Here's how the part is built. I have some questions about the finished solid (model axes, mm). A direction names the side the tool comes from. Give positions to 0.01 mm unless a question says otherwise; leave off trailing zeros. Loops run counter-clockwise (first coordinate to the right, second up) from the corner with the lowest first, then second, coordinate; pieces in that order, holes last. Notation, with made-up numbers: (19, 56.5) - (42, 56.5) arc R10 ccw to (42, 74.5) - close; hole circle Ø6 at (59, -12.5). An arc over 180 degrees is marked (long way). Use a Markdown table: item, result.
from build123d import *

# Parameters (mm, degrees)
SKETCH_1_W          = 42
SKETCH_1_H          = 42
EXTRUDE_1_DEPTH     = 5
SKETCH_2_R          = 17.5
CUT_EXTRUDE_1_DEPTH = 6
SKETCH_3_R          = 18.5
CUT_EXTRUDE_2_DEPTH = 4
SKETCH_4_R          = 19
CUT_EXTRUDE_3_DEPTH = 2
FILLET_1_R          = 4
SKETCH_5_R          = 1.6
CUT_EXTRUDE_4_DEPTH = 6
SKETCH_7_R          = 1.15
CUT_EXTRUDE_5_DEPTH = 6
SKETCH_8_R          = 2
CUT_EXTRUDE_6_DEPTH = 3


with BuildPart() as part:
    # 草图1 → 凸台-拉伸1 (new body)
    with BuildSketch(Plane.XY):
        Rectangle(SKETCH_1_W, SKETCH_1_H)
    extrude(amount=EXTRUDE_1_DEPTH)

    # 草图2 → 切除-拉伸1 (cut, through all)
    with BuildSketch(Plane.XY.offset(5)):
        Circle(SKETCH_2_R)
    extrude(amount=-CUT_EXTRUDE_1_DEPTH, mode=Mode.SUBTRACT)

    # 草图3 → 切除-拉伸2 (cut)
    with BuildSketch(Plane.XY.offset(5)):
        Circle(SKETCH_3_R)
    extrude(amount=-CUT_EXTRUDE_2_DEPTH, mode=Mode.SUBTRACT)

    # 草图4 → 切除-拉伸3 (cut)
    with BuildSketch(Plane.XY.offset(5)):
        Circle(SKETCH_4_R)
    extrude(amount=-CUT_EXTRUDE_3_DEPTH, mode=Mode.SUBTRACT)

    # 圆角1
    fillet_1_edges = [part.edges().sort_by_distance(p)[0] for p in [
        (21, -21, 2.5),
        (-21, -21, 2.5),
        (-21, 21, 2.5),
        (21, 21, 2.5),
    ]]
    fillet(fillet_1_edges, radius=FILLET_1_R)

    # 草图5 → 切除-拉伸4 (cut, through all)
    with BuildSketch(Plane.XY.offset(5)):
        with Locations((-16.970562748, 16.970562748)):
            Circle(SKETCH_5_R)
        with Locations((16.970562748, 16.970562748)):
            Circle(SKETCH_5_R)
        with Locations((16.970562748, -16.970562748)):
            Circle(SKETCH_5_R)
        with Locations((-16.970562748, -16.970562748)):
            Circle(SKETCH_5_R)
    extrude(amount=-CUT_EXTRUDE_4_DEPTH, mode=Mode.SUBTRACT)

    # 草图7 → 切除-拉伸5 (cut, through all)
    with BuildSketch(Plane(origin=(0, 0, 0), x_dir=(-1, 0, 0), z_dir=(0, 0, -1))):
        with Locations((-18, 12)):
            Circle(SKETCH_7_R)
        with Locations((18, 12)):
            Circle(SKETCH_7_R)
        with Locations((18, -12)):
            Circle(SKETCH_7_R)
        with Locations((-18, -12)):
            Circle(SKETCH_7_R)
    extrude(amount=-CUT_EXTRUDE_5_DEPTH, mode=Mode.SUBTRACT)

    # 草图8 → 切除-拉伸6 (cut)
    with BuildSketch(Plane(origin=(0, 0, 0), x_dir=(-1, 0, 0), z_dir=(0, 0, -1))):
        with Locations((-18, 12)):
            Circle(SKETCH_8_R)
        with Locations((18, 12)):
            Circle(SKETCH_8_R)
        with Locations((18, -12)):
            Circle(SKETCH_8_R)
        with Locations((-18, -12)):
            Circle(SKETCH_8_R)
    extrude(amount=-CUT_EXTRUDE_6_DEPTH, mode=Mode.SUBTRACT)


solid = part.part
(1) Suppose I cut it at A-A on x = 0. Write out the boundary of the cut face in (y, z).
A:
| item | result |
|---|---|
| outline | (-21, 0) - (-17.5, 0) - (-17.5, 1) - (-18.5, 1) - (-18.5, 3) - (-19, 3) - (-19, 5) - (-21, 5) - close; (17.5, 0) - (21, 0) - (21, 5) - (19, 5) - (19, 3) - (18.5, 3) - (18.5, 1) - (17.5, 1) - close |
(2) Will these pins go through, and if not, where does the flat tip stop? pin 1 (5 mm diameter, centred on x = 18, y = 12, fed in from -Z); pin 2 (1.2 mm diameter, centred on x = 17.5, y = 12, fed in from -Z) (3 decimals); pin 3 (3 mm diameter, centred on x = 18, y = 12, fed in from -Z).
A:
| item | result |
|---|---|
| pin 1 | z = 0 |
| pin 2 | through |
| pin 3 | z = 3 |
(3) Suppose I cut it at C-C on z = 4.45. Count the separate pieces of the cut face and the enclosed holes in it, plus the area to 3 significant figures.
A:
| item | result |
|---|---|
| separate pieces | 1 |
| enclosed holes | 9 |
| area | 567 mm2 |
(4) We'd pull the mould along X, two halves only. Please class faces 4 (the face through (0, 19, 0)), 5 (the face through (19.797, 19.859, 2.535)), 6 (the face through (4.1, -18.2, 3)): pulls with the +X half, pulls with the -X half, needs draft (parallel to the pull), parting line crosses it, or undercut.
A:
| item | result |
|---|---|
| face 4 | needs draft |
| face 5 | pulls with the +X half |
| face 6 | undercut |
(5) Suppose I cut it at B-B on y = -1.5. Write out the boundary of the cut face in (x, z), plus the area to 3 significant figures.
A:
| item | result |
|---|---|
| outline | (-21, 0) - (-17.44, 0) - (-17.44, 1) - (-18.44, 1) - (-18.44, 3) - (-18.94, 3) - (-18.94, 5) - (-21, 5) - close; (17.44, 0) - (21, 0) - (21, 5) - (18.94, 5) - (18.94, 3) - (18.44, 3) - (18.44, 1) - (17.44, 1) - close |
| area | 25.6 mm2 |
(6) On a 3-axis mill with a long thin cutter (end or side, diameter ignored), from which of +Z, -Z, +X, -X, +Y, -Y can I reach the whole of each face in a straight line? I mean faces 1 (the face through (-16.85, 12.05, 3.99)), 2 (the face through (-11, -14, 1)), 3 (the face through (-18, 14, 1)). Say none if no direction works.
A:
| item | result |
|---|---|
| face 1 | +Z, -Z |
| face 2 | +Z |
| face 3 | -Z |
(7) If I drill on line 1 (Y direction, x = 0, z = 1.85); line 2 (X direction, y = -6, z = 1.85); line 3 (Y direction, x = -4, z = 4.5), over which ranges is the centre line in solid material (lowest first)?
A:
| item | result |
|---|---|
| line 1 | -21 to -18.5, 18.5 to 21 |
| line 2 | -21 to -17.5, 17.5 to 21 |
| line 3 | -21 to -18.57, 18.57 to 21 |
